Study the drawing (mm; zero at the part's minimum x, y, z) and answer. A direction names the side the tool comes from. Coordinates: 2 decimals unless noted, no trailing zeros. Loops run counter-clockwise (first coordinate to the right, second up) from the corner with the lowest first, then second, coordinate; pieces in that order, holes last. Notation, with made-up numbers: (83, 28.5) -> (87, 28.5) arc R11 cw to (87, 34.5) -> close; hole circle Ø3 at (28.25, 30). An arc over 180 degrees is marked (long way). Answer as CSV lines item,"result".
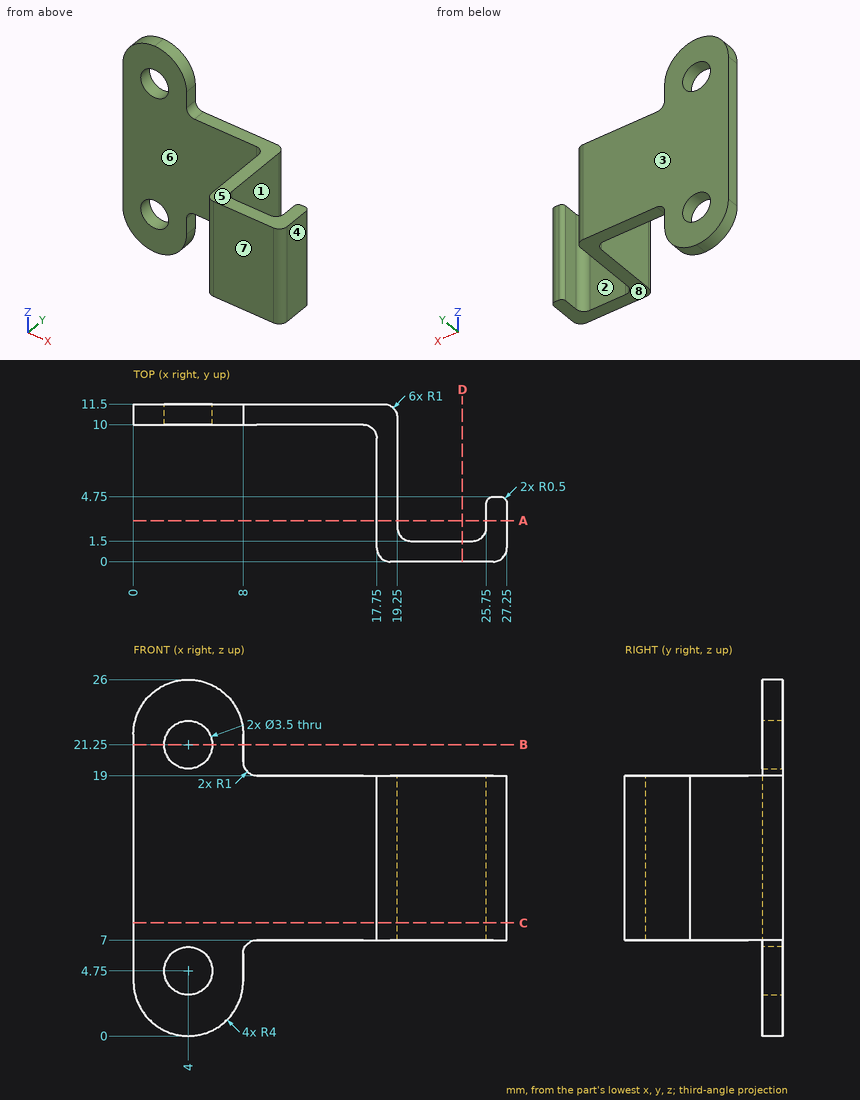
Q1. Find the intervals of material crossed by probe 1 along X at (y, z) = (10.75, 4.75); probe 2 along Y at (x, z) = (3.75, 14.75); probe 3 along X at (y, z) = (7.75, 17.5), in increasing order. Write a range as [from, to].
Results:
probe 1,"x = [0, 2.25], [5.75, 8]"
probe 2,"y = [10, 11.5]"
probe 3,"x = [17.75, 19.25]"
Q2. A cutting plane is placed at A-A, the plane y = 3. Write down the section's boundary in (x, z).
Results:
outline,"(17.75, 7) -> (19.25, 7) -> (19.25, 19) -> (17.75, 19) -> close; (25.75, 7) -> (27.25, 7) -> (27.25, 19) -> (25.75, 19) -> close"
Q3. A cutting plane is placed at D-D, the plane x = 24. Write down the section's boundary in (y, z), and give its area (3 significant figures).
Results:
outline,"(0, 7) -> (1.5, 7) -> (1.5, 19) -> (0, 19) -> close"
area,"18.0 mm²"
Q4. For the marked faces 5, 6, 7 and 8, determine the directions among +Z, -Z, +X, -X, +Y, -Y from which every point of the face is accessible in a straight line to the end or side of a thin tool.
Results:
face 5,"+Z, +X, +Y, -Y"
face 6,"+Z, -Z, -X, -Y"
face 7,"+Z, -Z, +X, -X, -Y"
face 8,"-Z, +X, +Y, -Y"
Q5. For a pull along X with two mould halves and no side action, classify the marked faces 1, 2, 3 and 4 as pulls with the +X half, pulls with the -X half, needs draft (parallel to the pull), parting line crosses it, or undercut.
Results:
face 1,"undercut"
face 2,"undercut"
face 3,"needs draft"
face 4,"pulls with the +X half"
Q6. A cutting plane is placed at B-B, the plane z = 21.25. Write down the section's boundary in (x, y), and give its area (3 significant figures).
Results:
outline,"(0, 10) -> (2.25, 10) -> (2.25, 11.5) -> (0, 11.5) -> close; (5.75, 10) -> (8, 10) -> (8, 11.5) -> (5.75, 11.5) -> close"
area,"6.75 mm²"
Q7. A cutting plane is placed at C-C, the plane z = 8.25. Write down the section's boundary in (x, y).
Results:
outline,"(0, 10) -> (16.75, 10) arc R1 cw to (17.75, 9) -> (17.75, 1) arc R1 ccw to (18.75, 0) -> (26.25, 0) arc R1 ccw to (27.25, 1) -> (27.25, 4.25) arc R0.5 ccw to (26.75, 4.75) -> (26.25, 4.75) arc R0.5 ccw to (25.75, 4.25) -> (25.75, 2.5) arc R1 cw to (24.75, 1.5) -> (20.25, 1.5) arc R1 cw to (19.25, 2.5) -> (19.25, 10.5) arc R1 ccw to (18.25, 11.5) -> (0, 11.5) -> close"
Q8. Given pin 1 Ø4 at (y, z) = (3.5, 14) entering from -X; pin 2 Ø1.3 at (x, z) = (23.5, 12.5) entering from +Y; pin 3 Ø8 at (x, z) = (12.5, 8) entering from -Y, each flat-ended and moving along its own axis, determine where each tip first touches the part or whether it passes through.
Results:
pin 1,"stops at x = 17.75"
pin 2,"stops at y = 1.5"
pin 3,"stops at y = 10"
